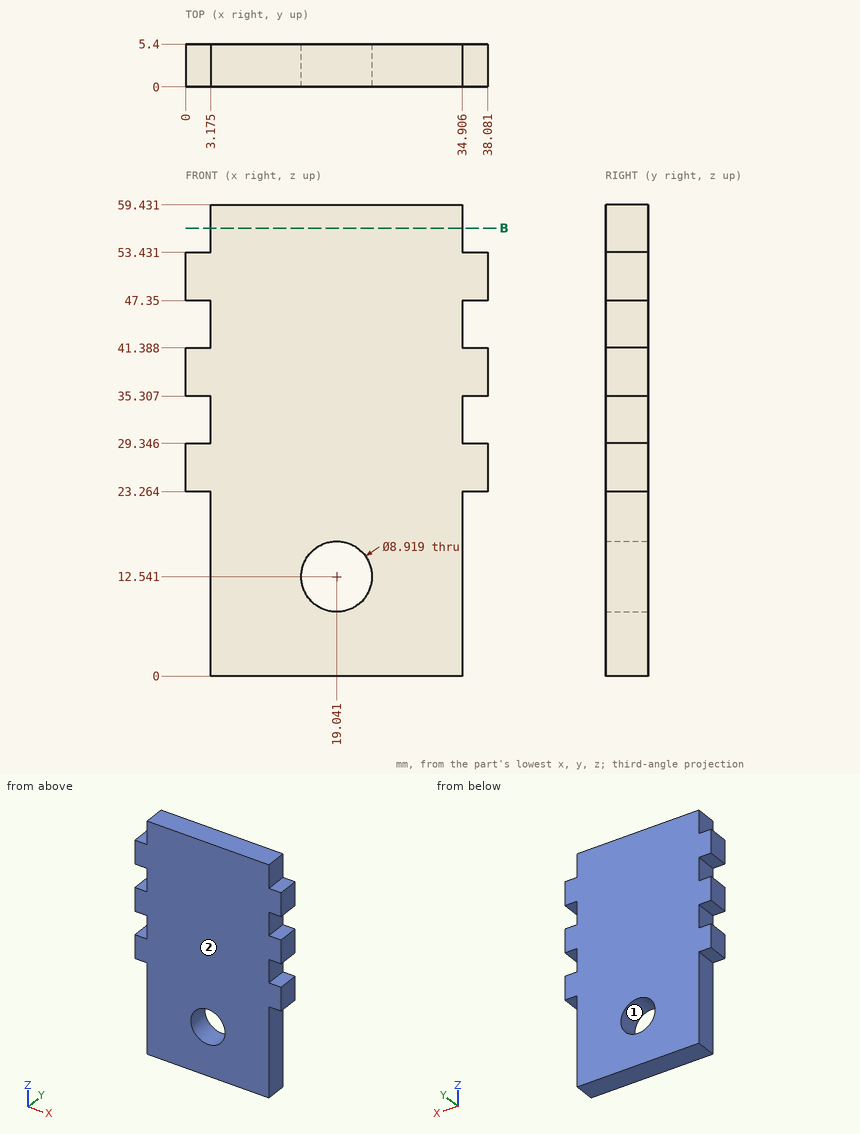
Part print with two shaded views. Sizes in mm from the minimum x, y, z corner. Give positions to 0.01 mm unless a question says otherwise; leave off trailing zeros. Order: outer loops, then holes, each group sorted by start corner. A loop starts at its lowest first (then second) coordinate and runs counter-clockwise, first axis right, second up.
1) Pin check, flat tips, straight feed: pin 1 (2 mm diameter, centred on y = 3.5, z = 11.5, fed in from -X) (3 decimals); pin 2 (1 mm diameter, centred on x = 2, y = 3.5, fed in from -Z); pin 3 (2 mm diameter, centred on y = 3, z = 16, fed in from +X). Stop position of each tip, or through.
2) Mould opens along X. For the marked faces 1 and 2 say: +X half, -X half, draft (parallel to the pull), parting line (faces both ways), or undercut.
3) Wall check: probe 1 along Z at (x, y) = (22, 3.7) (1 decimal); probe 2 along X at (y, z) = (4.45, 21.5) (1 decimal); probe 3 along Z at (x, y) = (16.5, 0.7) (1 decimal). Give the ranges that are in metal, low to high.
4) Saw through at B-B, the plane z = 56.5. Write the cut outline in (x, y) (1 decimal).
Computed:
1. pin 1: stops at x = 3.175
1. pin 2: stops at z = 23.26
1. pin 3: stops at x = 34.91
2. face 1: undercut
2. face 2: draft
3. probe 1: z = 0 to 9.2, 15.9 to 59.4
3. probe 2: x = 3.2 to 34.9
3. probe 3: z = 0 to 8.9, 16.2 to 59.4
4. outline: (3.2, 0) - (34.9, 0) - (34.9, 5.4) - (3.2, 5.4) - close
